```python
from build123d import *

# Parameters (mm, degrees)
BOSS_EXTRUDE1_DEPTH = 10
SKETCH2_R           = 1.445
BOSS_EXTRUDE2_DEPTH = 6
SKETCH4_R           = 1.45
CUT_EXTRUDE1_DEPTH  = 6


with BuildPart() as part:
    # Sketch1 → Boss-Extrude1 (new body)
    with BuildSketch(Plane(origin=(0, 0, 0), x_dir=(1, 0, 0), z_dir=(0, 1, 0))):
        Polygon((3.406366588, 0), (1.703183294, 2.95), (-1.703183294, 2.95), (-3.406366588, 0), (-1.703183294, -2.95), (1.703183294, -2.95), align=None)
    extrude(amount=BOSS_EXTRUDE1_DEPTH)

    # Sketch2 → Boss-Extrude2 (add)
    with BuildSketch(Plane.XZ):
        with Locations(Location((0, 0, 0), (0, 0, 90))):
            Circle(SKETCH2_R)
    extrude(amount=BOSS_EXTRUDE2_DEPTH)

    # Sketch4 → Cut-Extrude1 (cut)
    with BuildSketch(Plane(origin=(0, 10, 0), x_dir=(1, 0, 0), z_dir=(0, 1, 0))):
        with Locations(Location((0, 0, 0), (0, 0, 270))):
            Circle(SKETCH4_R)
    extrude(amount=-CUT_EXTRUDE1_DEPTH, mode=Mode.SUBTRACT)


solid = part.part
```
Check sheet for the modelled part. Datum: model origin and axes. Units: mm. A direction names the side the tool comes from. Give positions to 0.01 mm unless a question says otherwise; leave off trailing zeros. Write each loop counter-clockwise with the first axis right and the second up, starting at its lowest first coordinate (ties: lowest second). Pieces come first, ordered by that corner, then holes. Notation, with made-up numbers: (13, 67.25) - (59, 67.25) arc R26 cw to (59, 98.25) - close; hole circle Ø5 at (0.25, 82.5). An arc over 180 degrees is marked (long way). Answer as a JSON object with one key per item and string values. Group by question number.
1) Release check for a two-part mould opening along Z. For faces 1 (the face through (2.54, 4.93, 1.5)), 2 (the face through (0, 5, -2.95)), 3 (the face through (0.06, 7.04, -1.45)), 4 (the face through (1.5, 10, -0.7)) record: pulls with the +Z half, pulls with the -Z half, needs draft (parallel to the pull), parting line crosses it, or undercut.
2) Depth check by flat-ended pin: P1, Ø3, axis at y = 1, z = -2.5, coming from the -X side; P2, Ø1.5, axis at y = 4, z = -0.5, coming from the -X side; P3, Ø2.5, axis at x = 0, z = 0, coming from the +Y side. Enter the tip coordinate at first touch or a pass-through.
3) Sectioned sample at B-B (x = 0). Record the cut outline in (y, z) (3 decimals).
4) Thickness scan on probe 1 along Y at (x, z) = (-0.5, 0.1); probe 2 along Y at (x, z) = (-1.25, 2.65); probe 3 along X at (y, z) = (7.75, 1.25). Record the ranges inside material, lowest first. Write a range as from..to.
5) Sectioned sample at D-D (y = 3). Record the cut outline in (x, z).
6) Sectioned sample at A-A (y = 7.25). Record the cut outline in (x, z), then the cut area to 3 significant figures.
7) Access from +Z, -Z, +X, -X, +Y, -Y to the whole of each face (thin tool, end or side, straight path). Record for faces 5 (the face through (1.5, 0, -0.7)), 6 (the face through (0, 5, 2.95)), 7 (the face through (0, 4, 0)).
8) Sectioned sample at C-C (z = -0.85). Record the cut outline in (x, y).
Geometry results:
{
 "1": {"face 1": "pulls with the +Z half", "face 2": "pulls with the -Z half", "face 3": "undercut", "face 4": "needs draft"},
 "2": {"P1": "stops at x = -2.83", "P2": "stops at x = -3.41", "P3": "stops at y = 4"},
 "3": {"outline": "(-6, -1.445) - (0, -1.445) - (0, -2.95) - (10, -2.95) - (10, -1.45) - (4, -1.45) - (4, 1.45) - (10, 1.45) - (10, 2.95) - (0, 2.95) - (0, 1.445) - (-6, 1.445) - close"},
 "4": {"probe 1": "y = -6..4", "probe 2": "y = 0..10", "probe 3": "x = -2.68..-0.73, 0.73..2.68"},
 "5": {"outline": "(-3.41, 0) - (-1.7, -2.95) - (1.7, -2.95) - (3.41, 0) - (1.7, 2.95) - (-1.7, 2.95) - close"},
 "6": {"outline": "(-3.41, 0) - (-1.7, -2.95) - (1.7, -2.95) - (3.41, 0) - (1.7, 2.95) - (-1.7, 2.95) - close; hole circle Ø2.9 at (0, 0)", "area": "23.5 mm^2"},
 "7": {"face 5": "-Y", "face 6": "+Z, +X, -X, +Y, -Y", "face 7": "+Y"},
 "8": {"outline": "(-2.92, 0) - (-1.17, 0) - (-1.17, -6) - (1.17, -6) - (1.17, 0) - (2.92, 0) - (2.92, 10) - (1.17, 10) - (1.17, 4) - (-1.17, 4) - (-1.17, 10) - (-2.92, 10) - close"}
}
